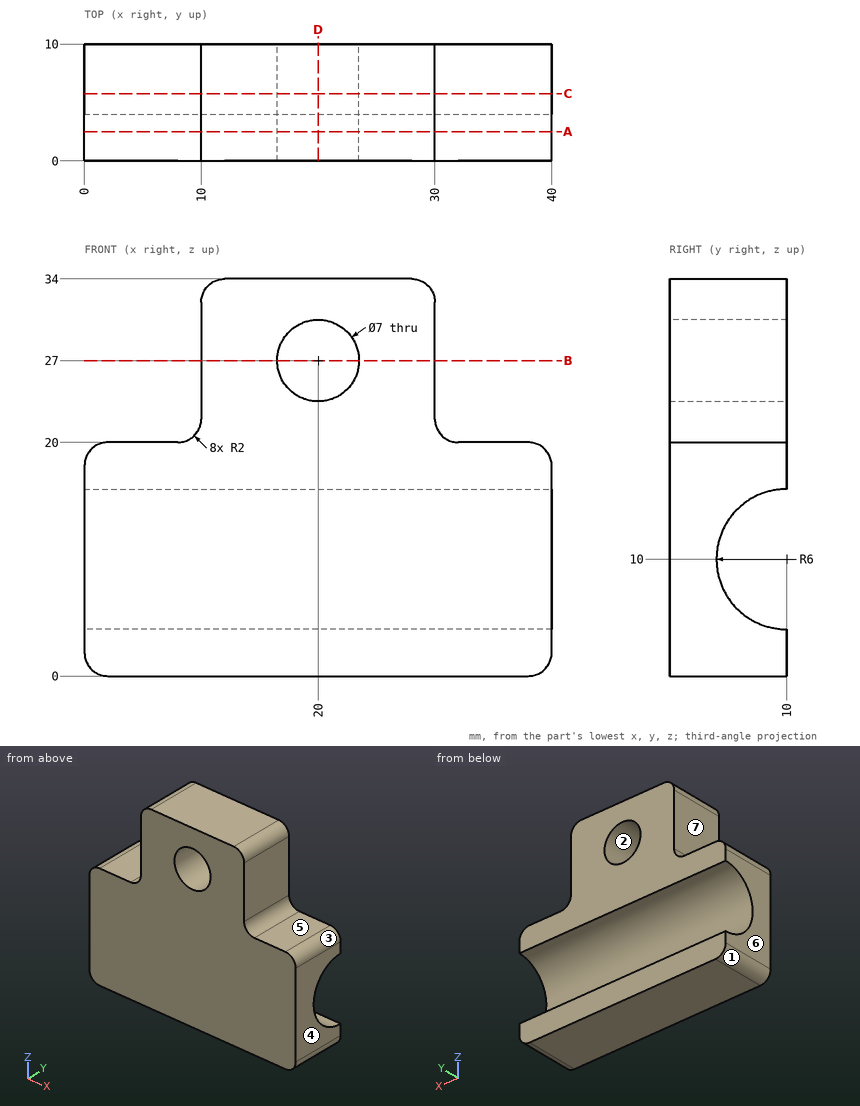
Input: dimensioned drawing with shaded views. Units: mm. Origin: part minimum x, y, z. A direction names the side the tool comes from. Coordinates: 2 decimals unless noted, no trailing zeros. Order: outer loops, then holes, each group sorted by start corner. A loop starts at its lowest first (then second) coordinate and runs counter-clockwise, first axis right, second up.
(1) First-contact query: pin 1 (6 mm diameter, centred on x = 9.5, z = 8.5, fed in from +Y); pin 2 (4 mm diameter, centred on x = 9.5, y = 6, fed in from +Z); pin 3 (3 mm diameter, centred on x = 35, y = 4.5, fed in from +Z); pin 4 (4 mm diameter, centred on x = 20, z = 27, fed in from +Y). Flat tips, straight axial feed; report the tip coordinate or a pass-through.
(2) Section query A-A (y = 2.5). Return the cut outline in (x, z).
(3) Access query for the marked faces 5, 6 and 7. Directions: +Z, -Z, +X, -X, +Y, -Y. A direction counts if a zero-diameter tool reaches every point of the face in a straight line with its end or side. Return the directions, or none.
(4) Section query B-B (z = 27). Return the cut outline in (x, y).
(5) Section query C-C (y = 5.75). Return the cut outline in (x, z).
(6) Material intervals for probe 1 along X at (y, z) = (7.75, 27); probe 2 along Z at (x, y) = (18.5, 6.75); probe 3 along Z at (x, y) = (26, 4.5), sorted ascending.
(7) Draft query along Z for the marked faces 1, 2, 3 and 4. Return one class per face: pulls with the +Z half, pulls with the -Z half, needs draft (parallel to the pull), parting line crosses it, or undercut.
(8) Section query D-D (x = 20). Return the cut outline in (y, z).
Solution:
1. pin 1: stops at y = 6.03
1. pin 2: stops at z = 33.94
1. pin 3: stops at z = 20
1. pin 4: passes through
2. outline: (0, 2) arc R2 ccw to (2, 0) - (38, 0) arc R2 ccw to (40, 2) - (40, 18) arc R2 ccw to (38, 20) - (32, 20) arc R2 cw to (30, 22) - (30, 32) arc R2 ccw to (28, 34) - (12, 34) arc R2 ccw to (10, 32) - (10, 22) arc R2 cw to (8, 20) - (2, 20) arc R2 ccw to (0, 18) - close; hole circle Ø7 at (20, 27)
3. face 5: +Z, +X, +Y, -Y
3. face 6: +Z, -Z, -X, +Y, -Y
3. face 7: +Z, -X, +Y, -Y
4. outline: (10, 0) - (16.5, 0) - (16.5, 10) - (10, 10) - close; (23.5, 0) - (30, 0) - (30, 10) - (23.5, 10) - close
5. outline: (0, 2) arc R2 ccw to (2, 0) - (38, 0) arc R2 ccw to (40, 2) - (40, 5.76) - (0, 5.76) - close; (0, 14.24) - (40, 14.24) - (40, 18) arc R2 ccw to (38, 20) - (32, 20) arc R2 cw to (30, 22) - (30, 32) arc R2 ccw to (28, 34) - (12, 34) arc R2 ccw to (10, 32) - (10, 22) arc R2 cw to (8, 20) - (2, 20) arc R2 ccw to (0, 18) - close; hole circle Ø7 at (20, 27)
6. probe 1: x = 10 to 16.5, 23.5 to 30
6. probe 2: z = 0 to 4.96, 15.04 to 23.84, 30.16 to 34
6. probe 3: z = 0 to 7.6, 12.4 to 34
7. face 1: pulls with the -Z half
7. face 2: undercut
7. face 3: pulls with the +Z half
7. face 4: needs draft
8. outline: (0, 0) - (10, 0) - (10, 4) arc R6 cw to (10, 16) - (10, 23.5) - (0, 23.5) - close; (0, 30.5) - (10, 30.5) - (10, 34) - (0, 34) - close
